from build123d import *

# Parameters (mm, degrees)
SZKIC1_W                    = 25
SZKIC1_H                    = 7
DODANIE_WYCI_GNI_CIE1_DEPTH = 3
SZKIC2_W                    = 15
SZKIC2_H                    = 32
DODANIE_WYCI_GNI_CIE2_DEPTH = 4
SZKIC3_R                    = 1.6
WYTNIJ_WYCI_GNI_CIE1_DEPTH  = 43.393985422
WYTNIJ_WYCI_GNI_CIE2_REACH  = 45.339
SZKIC4_W                    = 5.5
SZKIC4_H                    = 8
WYTNIJ_WYCI_GNI_CIE3_REACH  = 45.339
SZKIC5_R                    = 1.35
SFAZOWANIE1_SIZE            = 1.5
SFAZOWANIE2_SIZE            = 2


with BuildPart() as part:
    # Szkic1 → Dodanie-wyciągnięcie1 (new body)
    with BuildSketch(Plane.XY):
        with Locations((12.5, 0)):
            Rectangle(SZKIC1_W, SZKIC1_H)
    extrude(amount=DODANIE_WYCI_GNI_CIE1_DEPTH)

    # Szkic2 → Dodanie-wyciągnięcie2 (add)
    with BuildSketch(Plane(origin=(25, 0, 0), x_dir=(0, 0, -1), z_dir=(1, 0, 0))):
        with Locations((-7.5, 12.5)):
            Rectangle(SZKIC2_W, SZKIC2_H)
    extrude(amount=DODANIE_WYCI_GNI_CIE2_DEPTH)

    # Szkic3 → Wytnij-wyciągnięcie1 (cut, through all)
    with BuildSketch(Plane.XY.offset(3)):
        with Locations((5, 0)):
            Circle(SZKIC3_R)
        with Locations((20, 0)):
            Circle(SZKIC3_R)
    extrude(amount=-WYTNIJ_WYCI_GNI_CIE1_DEPTH, mode=Mode.SUBTRACT)

    # Szkic4 → Wytnij-wyciągnięcie2 (cut, up to next)
    with BuildSketch(Plane(origin=(29, 0, 0), x_dir=(0, 0, -1), z_dir=(1, 0, 0)), mode=Mode.PRIVATE) as wytnij_wyci_gni_cie2_sk1:
        with Locations((-2.75, 24.5)):
            Rectangle(SZKIC4_W, SZKIC4_H)
    wytnij_wyci_gni_cie2_tool1 = extrude(wytnij_wyci_gni_cie2_sk1.sketch, amount=-WYTNIJ_WYCI_GNI_CIE2_REACH, mode=Mode.PRIVATE) & part.part
    add(wytnij_wyci_gni_cie2_tool1.solids().sort_by_distance((29, 24.5, 2.75))[0], mode=Mode.SUBTRACT)

    # Szkic5 → Wytnij-wyciągnięcie3 (cut, up to next)
    with BuildSketch(Plane(origin=(29, 0, 0), x_dir=(0, 0, -1), z_dir=(1, 0, 0)), mode=Mode.PRIVATE) as wytnij_wyci_gni_cie3_sk1:
        with Locations((-11, 12.5)):
            Circle(SZKIC5_R)
    wytnij_wyci_gni_cie3_tool1 = extrude(wytnij_wyci_gni_cie3_sk1.sketch, amount=-WYTNIJ_WYCI_GNI_CIE3_REACH, mode=Mode.PRIVATE) & part.part
    # Szkic5 → Wytnij-wyciągnięcie3 (cut, up to next)
    with BuildSketch(Plane(origin=(29, 0, 0), x_dir=(0, 0, -1), z_dir=(1, 0, 0)), mode=Mode.PRIVATE) as wytnij_wyci_gni_cie3_sk2:
        with Locations((-4, 12.5)):
            Circle(SZKIC5_R)
    wytnij_wyci_gni_cie3_tool2 = extrude(wytnij_wyci_gni_cie3_sk2.sketch, amount=-WYTNIJ_WYCI_GNI_CIE3_REACH, mode=Mode.PRIVATE) & part.part
    # Szkic5 → Wytnij-wyciągnięcie3 (cut, up to next)
    with BuildSketch(Plane(origin=(29, 0, 0), x_dir=(0, 0, -1), z_dir=(1, 0, 0)), mode=Mode.PRIVATE) as wytnij_wyci_gni_cie3_sk3:
        with Locations((-11, 5.5)):
            Circle(SZKIC5_R)
    wytnij_wyci_gni_cie3_tool3 = extrude(wytnij_wyci_gni_cie3_sk3.sketch, amount=-WYTNIJ_WYCI_GNI_CIE3_REACH, mode=Mode.PRIVATE) & part.part
    # Szkic5 → Wytnij-wyciągnięcie3 (cut, up to next)
    with BuildSketch(Plane(origin=(29, 0, 0), x_dir=(0, 0, -1), z_dir=(1, 0, 0)), mode=Mode.PRIVATE) as wytnij_wyci_gni_cie3_sk4:
        with Locations((-11, 19.5)):
            Circle(SZKIC5_R)
    wytnij_wyci_gni_cie3_tool4 = extrude(wytnij_wyci_gni_cie3_sk4.sketch, amount=-WYTNIJ_WYCI_GNI_CIE3_REACH, mode=Mode.PRIVATE) & part.part
    add(wytnij_wyci_gni_cie3_tool1.solids().sort_by_distance((29, 12.5, 11))[0], mode=Mode.SUBTRACT)
    add(wytnij_wyci_gni_cie3_tool2.solids().sort_by_distance((29, 12.5, 4))[0], mode=Mode.SUBTRACT)
    add(wytnij_wyci_gni_cie3_tool3.solids().sort_by_distance((29, 5.5, 11))[0], mode=Mode.SUBTRACT)
    add(wytnij_wyci_gni_cie3_tool4.solids().sort_by_distance((29, 19.5, 11))[0], mode=Mode.SUBTRACT)

    # Sfazowanie1
    sfazowanie1_edges = [part.edges().sort_by_distance(p)[0] for p in [
        (29, -3.5, 7.5),
        (29, 28.5, 10.25),
        (27, 20.5, 5.5),
    ]]
    chamfer(sfazowanie1_edges, length=SFAZOWANIE1_SIZE)

    # Sfazowanie2
    sfazowanie2_edges = [part.edges().sort_by_distance(p)[0] for p in [
        (25, 0, 3),
    ]]
    chamfer(sfazowanie2_edges, length=SFAZOWANIE2_SIZE)


solid = part.part
Read the model definition and answer for the solid it produces. Units are mm, in the model's axes. A direction names the side the tool comes from. Coordinates: 2 decimals unless noted, no trailing zeros. Loops run counter-clockwise (first coordinate to the right, second up) from the corner with the lowest first, then second, coordinate; pieces in that order, holes last. Notation, with made-up numbers: (37.25, 42) - (96.25, 42) arc R11 ccw to (96.25, 53) - close; hole circle Ø3 at (8, 61.5). An arc over 180 degrees is marked (long way). Answer in a Markdown table with one row per item.
Q1. Find section C-C on y = 5.5. Write down the section's boundary in (x, z).
Here are the results:
| item | result |
|---|---|
| outline | (25, 0) - (29, 0) - (29, 9.65) - (25, 9.65) - close; (25, 12.35) - (29, 12.35) - (29, 15) - (25, 15) - close |
Q2. Find section A-A on x = 20. Write down the section's boundary in (y, z).
Here are the results:
| item | result |
|---|---|
| outline | (-3.5, 0) - (-1.6, 0) - (-1.6, 3) - (-3.5, 3) - close; (1.6, 0) - (3.5, 0) - (3.5, 3) - (1.6, 3) - close |
Q3. For faces 4 (the flat face through (27, 20.5, 2)), 5 (the flat face through (11, 0, 3)), 6 (the flat face through (29, 13, 8)), 7 (the flat face through (12, 3.5, 1)), 8 (the flat face through (25, 13, 8)), determine the directions among +Z, -Z, +X, -X, +Y, -Y from which every point of the face is accessible in a straight line to the end or side of a thin tool.
Here are the results:
| item | result |
|---|---|
| face 4 | -Z, +X, -X, +Y |
| face 5 | +Z, -X, +Y, -Y |
| face 6 | +Z, -Z, +X, +Y, -Y |
| face 7 | +Z, -Z, -X, +Y |
| face 8 | +Z, -X, +Y |
Q4. Find section D-D on y = 0. Write down the section's boundary in (x, z), plus the area to 3 significant figures.
Here are the results:
| item | result |
|---|---|
| outline | (0, 0) - (3.4, 0) - (3.4, 3) - (0, 3) - close; (6.6, 0) - (18.4, 0) - (18.4, 3) - (6.6, 3) - close; (21.6, 0) - (29, 0) - (29, 15) - (25, 15) - (25, 5) - (23, 3) - (21.6, 3) - close |
| area | 118 mm^2 |
Q5. Given P1, Ø5.5, axis at x = 15.5, z = 3, coming from the +Y side; P2, Ø2, axis at x = 28, z = 1.5, coming from the +Y side; P3, Ø1.5, axis at y = 15, z = 12.5, coming from the -X side, each flat-ended and moving along its own axis, determine where each tip first touches the part or whether it passes through.
Here are the results:
| item | result |
|---|---|
| P1 | stops at y = 3.5 |
| P2 | stops at y = 20.5 |
| P3 | stops at x = 25 |
Q6. Straight lines are drawn through the part: line 1 along Y through (x, z) = (27.65, 11); line 2 along Y through (x, z) = (26.85, 11); line 3 along X through (y, z) = (20, 12.5). For each, find the intervals that lie inside material, in ascending order. Write a range as [from, to].
Here are the results:
| item | result |
|---|---|
| line 1 | y = [-3.35, 4.15], [6.85, 11.15], [13.85, 18.15], [20.85, 28.35] |
| line 2 | y = [-3.5, 4.15], [6.85, 11.15], [13.85, 18.15], [20.85, 28.5] |
| line 3 | x = [25, 29] |
Q7. Find section B-B on z = 11. Write down the section's boundary in (x, y), plus the area to 4 significant figures.
Here are the results:
| item | result |
|---|---|
| outline | (25, -3.5) - (27.5, -3.5) - (29, -2) - (29, 4.15) - (25, 4.15) - close; (25, 6.85) - (29, 6.85) - (29, 11.15) - (25, 11.15) - close; (25, 13.85) - (29, 13.85) - (29, 18.15) - (25, 18.15) - close; (25, 20.85) - (29, 20.85) - (29, 27) - (27.5, 28.5) - (25, 28.5) - close |
| area | 93.35 mm^2 |
Q8. The mould has two halves that part along X. Classify faces 1 (the flat face through (26, 28.5, 10)), 2 (the cylindrical face through (18.82, 1.08, 1.52)), 3 (the flat face through (0, 0, 1)): pulls with the +X half, pulls with the -X half, needs draft (parallel to the pull), parting line crosses it, or undercut.
Here are the results:
| item | result |
|---|---|
| face 1 | needs draft |
| face 2 | undercut |
| face 3 | pulls with the -X half |
